The drawing under review shows one solid part. Ordinate dimensions are in mm from its lowest x, y, z. A direction names the side the tool comes from. Give positions to 0.01 mm unless a question says otherwise; leave off trailing zeros. Write each loop counter-clockwise with the first axis right and the second up, starting at its lowest first coordinate (ties: lowest second). Pieces come first, ordered by that corner, then holes.
Q1. We need section D-D (x = 27.5). Write out the cut boundary in (y, z), then the cut area to 3 significant figures.
Q2. For line 1 (X direction, y = 22.5, z = 6); line 2 (Y direction, x = 10.5, z = 9.25); line 3 (Y direction, x = 45, z = 9.5), list the stretches that pass through material, from the lowest coordinate up.
Q3. We need section B-B (y = 19). Write out the cut boundary in (x, z).
Q4. Insertion check: P1, Ø5, axis at x = 64.5, y = 58, coming from the +Z side. The pin has a flat end and moves straight along its axis. Give the tip position at first contact, or say it passes through.
Q5. Machinability: for the marked faces 1 and 2, which of the approach directions +Z, -Z, +X, -X, +Y, -Y give a long, thin tool a straight path to every point of the face, cutting with its end or side? Answer none if there is none.
Q6. Mouldability with a two-part tool opening along Y and no side actions: class the marked faces 3, 4 and 5 as released by +Y, released by -Y, zero draft, split by the parting line, or undercut.
Q7. We need section C-C (z = 11.5). Write out the cut boundary in (x, y).
Q8. We need section A-A (x = 64.5). Write out the cut boundary in (y, z).
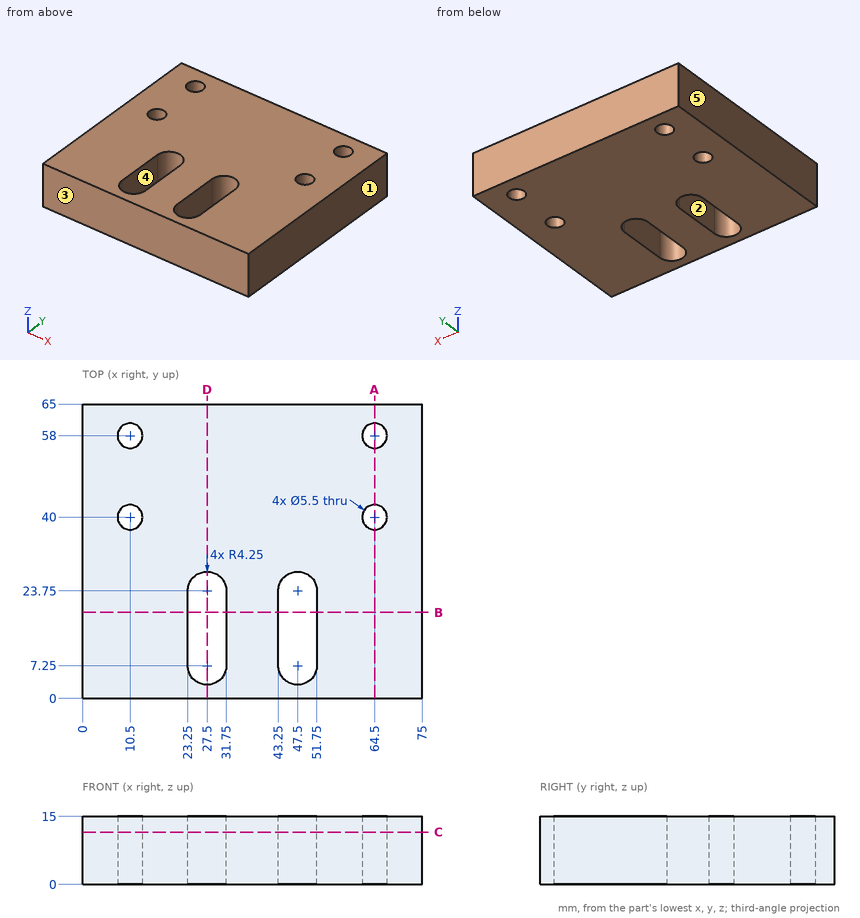
Computed:
1. outline: (0, 0) - (3, 0) - (3, 15) - (0, 15) - close; (28, 0) - (65, 0) - (65, 15) - (28, 15) - close
1. area: 600 mm2
2. line 1: x = 0 to 23.25, 31.75 to 43.25, 51.75 to 75
2. line 2: y = 0 to 37.25, 42.75 to 55.25, 60.75 to 65
2. line 3: y = 0 to 3.81, 27.19 to 65
3. outline: (0, 0) - (23.25, 0) - (23.25, 15) - (0, 15) - close; (31.75, 0) - (43.25, 0) - (43.25, 15) - (31.75, 15) - close; (51.75, 0) - (75, 0) - (75, 15) - (51.75, 15) - close
4. P1: passes through
5. face 1: +Z, -Z, +X, +Y, -Y
5. face 2: +Z, -Z
6. face 3: released by -Y
6. face 4: undercut
6. face 5: zero draft
7. outline: (0, 0) - (75, 0) - (75, 65) - (0, 65) - close; hole circle Ø5.5 at (10.5, 40); hole circle Ø5.5 at (10.5, 58); hole (23.25, 7.25) arc R4.25 ccw to (31.75, 7.25) - (31.75, 23.75) arc R4.25 ccw to (23.25, 23.75) - close; hole (43.25, 7.25) arc R4.25 ccw to (51.75, 7.25) - (51.75, 23.75) arc R4.25 ccw to (43.25, 23.75) - close; hole circle Ø5.5 at (64.5, 40); hole circle Ø5.5 at (64.5, 58)
8. outline: (0, 0) - (37.25, 0) - (37.25, 15) - (0, 15) - close; (42.75, 0) - (55.25, 0) - (55.25, 15) - (42.75, 15) - close; (60.75, 0) - (65, 0) - (65, 15) - (60.75, 15) - close
